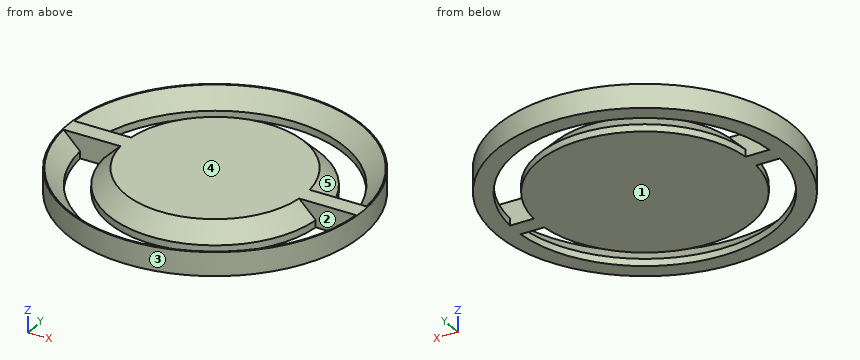
```python
from build123d import *

# Parameters (mm, degrees)
SKETCH_R        = 12.5
PAD_DEPTH       = 2
CHAMFER_SIZE    = 1.4
CHAMFER001_SIZE = 1.4


with BuildPart() as part:
    # Sketch (on XY_Plane of Origin) → Pad (new body)
    with BuildSketch(Plane.XY):
        Circle(SKETCH_R)
        with BuildLine():
            ThreePointArc((-8.968696, -0.75), (0, -9), (8.968696, -0.75))
            Line((8.968696, -0.75), (10.974402, -0.75))
            ThreePointArc((-10.974402, -0.75), (0, -11), (10.974402, -0.75))
            Line((-10.974402, -0.75), (-8.968696, -0.75))
        make_face(mode=Mode.SUBTRACT)
        with BuildLine():
            Line((-10.974402, 0.75), (-8.968696, 0.75))
            ThreePointArc((8.968696, 0.75), (0, 9), (-8.968696, 0.75))
            Line((8.968696, 0.75), (10.974402, 0.75))
            ThreePointArc((10.974402, 0.75), (0, 11), (-10.974402, 0.75))
        make_face(mode=Mode.SUBTRACT)
    extrude(amount=PAD_DEPTH)

    # Chamfer
    chamfer_edges = [part.edges().sort_by_distance(p)[0] for p in [
        (0, -9, 2),
        (0, 9, 2),
    ]]
    chamfer(chamfer_edges, length=CHAMFER_SIZE)

    # Chamfer001
    chamfer001_edges = [part.edges().sort_by_distance(p)[0] for p in [
        (0, -11, 2),
        (0, 11, 2),
    ]]
    chamfer(chamfer001_edges, length=CHAMFER001_SIZE)


solid = part.part
```
Verification items for the finished model (mm, model axes). Face numbers are marked on the shaded views. A direction names the side the tool comes from. Give positions to 0.01 mm unless a question says otherwise; leave off trailing zeros. Order: outer loops, then holes, each group sorted by start corner. A loop starts at its lowest first (then second) coordinate and runs counter-clockwise, first axis right, second up. Notation, with made-up numbers: (84, 69.25) -> (124, 69.25) arc R16 cw to (124, 99.25) -> close; hole circle Ø4 at (-19.75, 18.25). An arc over 180 degrees is marked (long way). One line per item, written item: value.
(1) Sectioned sample at A-A on x = 0. Record the cut outline in (y, z).
Final values:
outline: (-12.5, 0) -> (-11, 0) -> (-11, 0.6) -> (-12.4, 2) -> (-12.5, 2) -> close; (-9, 0) -> (9, 0) -> (9, 0.6) -> (7.6, 2) -> (-7.6, 2) -> (-9, 0.6) -> close; (11, 0) -> (12.5, 0) -> (12.5, 2) -> (12.4, 2) -> (11, 0.6) -> close
(2) Gauge pin test, flat ends, axial feed: pin 1 (0.6 mm diameter, centred on x = 9, z = 1.5, fed in from +Y); pin 2 (10 mm diameter, centred on x = -0.5, y = -6, fed in from -Z); pin 3 (0.6 mm diameter, centred on x = 9.5, z = 1, fed in from -Y); pin 4 (1 mm diameter, centred on x = -10, z = 1.5, fed in from +Y). Record the tip position at first contact, or that the pin passes through.
Final values:
pin 1: y = 8.98
pin 2: z = 0
pin 3: y = -8.46
pin 4: y = 8.12
(3) Scan lines: line 1 along X through (y, z) = (-4.75, 1); line 2 along X through (y, z) = (-4.5, 1.8); line 3 along Y through (x, z) = (-0.25, 1.7). Record each from-to range of solid material in increasing order. Write a range as [from, to].
Final values:
line 1: [-11.56, -10.36], [-7.17, 7.17], [10.36, 11.56]
line 2: [-11.66, -11.34], [-6.37, 6.37], [11.34, 11.66]
line 3: [-12.5, -12.1], [-7.9, 7.9], [12.1, 12.5]
(4) Sectioned sample at B-B on z = 1.35. Record the cut outline in (x, y), then the cut area to 3 significant figures.
Final values:
outline: circle Ø25 at (0, 0); hole (-11.73, -0.75) arc R11.75 ccw to (11.73, -0.75) -> (8.22, -0.75) arc R8.25 cw to (-8.22, -0.75) -> close; hole (-11.73, 0.75) -> (-8.22, 0.75) arc R8.25 cw to (8.22, 0.75) -> (11.73, 0.75) arc R11.75 ccw to start
area: 281 mm^2
(5) Tool access check on the marked faces 4 and 5. Record the directions out of +Z, -Z, +X, -X, +Y, -Y that give a thin tool (end or side, any length) a straight path to the whole face; none if there is none.
Final values:
face 4: +Z, +X, -X, +Y, -Y
face 5: +Z
(6) Draft check along Y on the marked faces 1, 2 and 3. Enter one of: pulls with the +Y half, pulls with the -Y half, needs draft (parallel to the pull), parting line crosses it, or undercut.
Final values:
face 1: needs draft
face 2: undercut
face 3: parting line crosses it
(7) Sectioned sample at C-C on y = -7. Count the separate pieces of the cut face and the enclosed holes in it, then the cut area to 3 significant figures.
Final values:
separate pieces: 3
enclosed holes: 0
area: 24.1 mm^2
